CAD build for the part. Positions are in the model's coordinates, mm. A direction names the side the tool comes from. Give positions to 0.01 mm unless a question says otherwise; leave off trailing zeros. Loops run counter-clockwise (first coordinate to the right, second up) from the corner with the lowest first, then second, coordinate; pieces in that order, holes last. Notation, with made-up numbers: M -30,60 L -19,60 A19 ccw -19,97 Z; hole C 53,86 d5. An arc over 180 degrees is marked long. Answer as CSV lines item,"result".
```python
from build123d import *

# Parameters (mm, degrees)
BOSS_EXTRUDE1_DEPTH = 3.175
SKETCH4_R           = 1.524
CUT_EXTRUDE1_DEPTH  = 4.175
CUT_EXTRUDE2_DEPTH  = 4.175


with BuildPart() as part:
    # Sketch1 → Boss-Extrude1 (new body)
    with BuildSketch(Plane.XY):
        Polygon((-3.81, 95.25), (-3.81, 0), (2.00025, 0), (2.00025, -3.175), (9.17575, -3.175), (9.17575, 0), (12.573, 0), (12.573, 5.588), (10.541, 5.588), (10.541, 8.128), (12.573, 8.128), (12.573, 15.748), (15.367, 15.748), (15.367, 8.128), (17.399, 8.128), (17.399, 5.588), (15.367, 5.588), (15.367, 0), (24.35225, 0), (24.35225, -3.175), (31.52775, -3.175), (31.52775, 0), (40.513, 0), (40.513, 5.588), (38.481, 5.588), (38.481, 8.128), (40.513, 8.128), (40.513, 15.748), (43.307, 15.748), (43.307, 8.128), (45.339, 8.128), (45.339, 5.588), (43.307, 5.588), (43.307, 0), (52.29225, 0), (52.29225, -3.175), (59.46775, -3.175), (59.46775, 0), (69.85, 0), (69.85, 95.25), (57.277, 95.25), (57.277, 88.646), (59.309, 88.646), (59.309, 86.106), (57.277, 86.106), (57.277, 78.486), (54.483, 78.486), (54.483, 86.106), (52.451, 86.106), (52.451, 88.646), (54.483, 88.646), (54.483, 95.25), (45.49775, 95.25), (45.49775, 98.425), (38.32225, 98.425), (38.32225, 95.25), (29.337, 95.25), (29.337, 88.646), (31.369, 88.646), (31.369, 86.106), (29.337, 86.106), (29.337, 78.486), (26.543, 78.486), (26.543, 86.106), (24.511, 86.106), (24.511, 88.646), (26.543, 88.646), (26.543, 95.25), (17.55775, 95.25), (17.55775, 98.425), (10.38225, 98.425), (10.38225, 95.25), align=None)
    extrude(amount=BOSS_EXTRUDE1_DEPTH)

    # Sketch4 → Cut-Extrude1 (cut, through all)
    with BuildSketch(Plane.XY.offset(3.175)):
        with Locations((66.04, 68.326)):
            Circle(SKETCH4_R)
        with Locations((66.04, 78.486)):
            Circle(SKETCH4_R)
    extrude(amount=-CUT_EXTRUDE1_DEPTH, mode=Mode.SUBTRACT)

    # Sketch5 → Cut-Extrude2 (cut, through all)
    with BuildSketch(Plane.XY.offset(3.175)):
        Polygon((12.237024548, 46.228), (12.237024548, 49.022), (5.061524548, 49.022), (5.061524548, 47.625), (5.061524548, 46.228), align=None)
        with BuildLine():
            ThreePointArc((21.730274548, 47.625), (20.206274548, 49.149), (18.682274548, 47.625))
            Line((18.682274548, 47.625), (20.206274548, 47.625))
            Line((20.206274548, 47.625), (21.730274548, 47.625))
        make_face()
        with BuildLine():
            Line((20.206274548, 47.625), (18.682274548, 47.625))
            ThreePointArc((18.682274548, 47.625), (20.206274548, 46.101), (21.730274548, 47.625))
            Line((21.730274548, 47.625), (20.206274548, 47.625))
        make_face()
        Polygon((28.175524548, 46.228), (28.175524548, 47.625), (28.175524548, 49.022), (35.351024548, 49.022), (35.351024548, 46.228), align=None)
        with BuildLine():
            ThreePointArc((44.844274548, 47.625), (43.320274548, 49.149), (41.796274548, 47.625))
            Line((41.796274548, 47.625), (43.320274548, 47.625))
            Line((43.320274548, 47.625), (44.844274548, 47.625))
        make_face()
        with BuildLine():
            Line((43.320274548, 47.625), (41.796274548, 47.625))
            ThreePointArc((41.796274548, 47.625), (43.320274548, 46.101), (44.844274548, 47.625))
            Line((44.844274548, 47.625), (43.320274548, 47.625))
        make_face()
        Polygon((51.289524548, 46.228), (51.289524548, 47.625), (51.289524548, 49.022), (58.465024548, 49.022), (58.465024548, 46.228), align=None)
    extrude(amount=-CUT_EXTRUDE2_DEPTH, mode=Mode.SUBTRACT)


solid = part.part
```
Q1. Wall check: line 1 (X direction, y = 13, z = 2.35); line 2 (Y direction, x = 53.5, z = 1.5) (3 decimals); line 3 (X direction, y = 84, z = 2.35). Give the ranges that are in metal, low to high. Write a range as [from, to].
Solution:
line 1,"x = [-3.81, 12.57], [15.37, 40.51], [43.31, 69.85]"
line 2,"y = [-3.175, 46.228], [49.022, 86.106], [88.646, 95.25]"
line 3,"x = [-3.81, 26.54], [29.34, 54.48], [57.28, 69.85]"
Q2. Pin check, flat tips, straight feed: P1, Ø0.6, axis at x = 12, z = 1.5, coming from the -Y side; P2, Ø1.8, axis at x = 66.04, y = 68.326, coming from the -Z side; P3, Ø1, axis at x = 55.5, z = 3, coming from the +Y side; P4, Ø1.6, axis at y = -1, z = 1, coming from the +X side. Stop position of each tip, or through.
Solution:
P1,"stops at y = 0"
P2,"passes through"
P3,"stops at y = 78.49"
P4,"stops at x = 59.47"
Q3. Cut at C-C (z = 1.5). Give the number of separate pieces and of enclosed holes in the cut face, and give its area (3 significant figures).
Solution:
separate pieces,"1"
enclosed holes,"7"
area,"6,820 mm²"
Q4. Which spindle directions (+Z, -Z, +X, -X, +Y, -Y) get a long thin tool onto all of the face, cutting with end or side? Do faces 1 (the flat face through (40.513, 3, 2)), 2 (the flat face through (50, 95.25, 2)), 3 (the flat face through (9, 46.228, 2)), 4 (the flat face through (54.483, 92, 2)). Say none if no direction does.
Solution:
face 1,"+Z, -Z, -Y"
face 2,"+Z, -Z, +X, +Y"
face 3,"+Z, -Z"
face 4,"+Z, -Z, +Y"
Q5. Cut at A-A (y = 9.5). Write the cut outline in (x, z) (3 decimals), and give its area (3 significant figures).
Solution:
outline,"M -3.81,0 L 12.573,0 L 12.573,3.175 L -3.81,3.175 Z; M 15.367,0 L 40.513,0 L 40.513,3.175 L 15.367,3.175 Z; M 43.307,0 L 69.85,0 L 69.85,3.175 L 43.307,3.175 Z"
area,"216 mm²"
Q6. Mould opens along X. For faces 5 (the flat face through (56, -3.175, 2)), 6 (the flat face through (29.337, 92, 2)) say: released by +X, released by -X, zero draft, split by the parting line, or undercut.
Solution:
face 5,"zero draft"
face 6,"undercut"
Q7. Cut at B-B (x = 66.04). Write the cut outline in (y, z) (3 decimals).
Solution:
outline,"M 0,0 L 66.802,0 L 66.802,3.175 L 0,3.175 Z; M 69.85,0 L 76.962,0 L 76.962,3.175 L 69.85,3.175 Z; M 80.01,0 L 95.25,0 L 95.25,3.175 L 80.01,3.175 Z"
